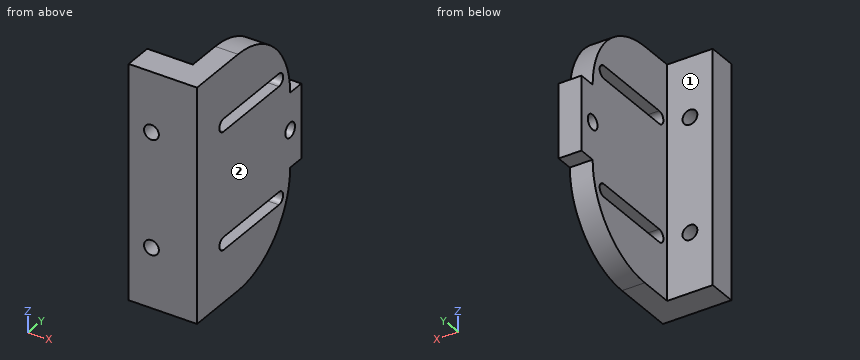
from build123d import *

# Parameters (mm, degrees)
SKETCH1_W           = 15.24
SKETCH1_H           = 52.07
BOSS_EXTRUDE1_DEPTH = 6.35
SKETCH2_W           = 5.08
SKETCH2_H           = 52.07
BOSS_EXTRUDE2_DEPTH = 25.4
CUT_EXTRUDE1_DEPTH  = 8.382
SKETCH4_R           = 1.651
CUT_EXTRUDE2_DEPTH  = 8.382
FILLET1_R           = 17.78
SKETCH6_W           = 5.08
SKETCH6_H           = 16.51
BOSS_EXTRUDE3_DEPTH = 3.81
SKETCH7_R           = 1.651
CUT_EXTRUDE3_DEPTH  = 14.478


with BuildPart() as part:
    # Sketch1 → Boss-Extrude1 (new body)
    with BuildSketch(Plane(origin=(0, 0, 0), x_dir=(1, 0, 0), z_dir=(0, 1, 0))):
        with Locations((7.62, 26.035)):
            Rectangle(SKETCH1_W, SKETCH1_H)
    extrude(amount=BOSS_EXTRUDE1_DEPTH)

    # Sketch2 → Boss-Extrude2 (add)
    with BuildSketch(Plane(origin=(0, 6.35, 0), x_dir=(1, 0, 0), z_dir=(0, 1, 0))):
        with Locations((12.7, 26.035)):
            Rectangle(SKETCH2_W, SKETCH2_H)
    extrude(amount=BOSS_EXTRUDE2_DEPTH)

    # Sketch3 → Cut-Extrude1 (cut)
    with BuildSketch(Plane(origin=(15.24, 0, 0), x_dir=(0, 0, -1), z_dir=(1, 0, 0))):
        with BuildLine():
            Line((14.4399, 27.94), (14.4399, 9.0424))
            ThreePointArc((14.4399, 9.0424), (13.0175, 7.62), (11.5951, 9.0424))
            Line((11.5951, 9.0424), (11.5951, 27.94))
            ThreePointArc((11.5951, 27.94), (13.0175, 29.3624), (14.4399, 27.94))
        make_face()
        with BuildLine():
            Line((40.50522627, 27.94), (40.50522627, 9.0424))
            ThreePointArc((40.50522627, 9.0424), (39.08282627, 7.62), (37.66042627, 9.0424))
            Line((37.66042627, 9.0424), (37.66042627, 27.94))
            ThreePointArc((37.66042627, 27.94), (39.08282627, 29.3624), (40.50522627, 27.94))
        make_face()
    extrude(amount=-CUT_EXTRUDE1_DEPTH, mode=Mode.SUBTRACT)

    # Sketch4 → Cut-Extrude2 (cut)
    with BuildSketch(Plane(origin=(0, 6.35, 0), x_dir=(1, 0, 0), z_dir=(0, 1, 0))):
        with Locations(Location((5.08, 38.735, 0), (0, 0, 270))):
            Circle(SKETCH4_R)
        with Locations(Location((5.08, 13.335, 0), (0, 0, 270))):
            Circle(SKETCH4_R)
    extrude(amount=-CUT_EXTRUDE2_DEPTH, mode=Mode.SUBTRACT)

    # Fillet1
    fillet1_edges = [part.edges().sort_by_distance(p)[0] for p in [
        (12.7, 31.75, -52.07),
        (12.7, 31.75, 0),
    ]]
    fillet(fillet1_edges, radius=FILLET1_R)

    # Sketch6 → Boss-Extrude3 (add)
    with BuildSketch(Plane(origin=(0, 31.75, 0), x_dir=(1, 0, 0), z_dir=(0, 1, 0))):
        with Locations((12.7, 26.035)):
            Rectangle(SKETCH6_W, SKETCH6_H)
    extrude(amount=BOSS_EXTRUDE3_DEPTH)

    # Sketch7 → Cut-Extrude3 (cut)
    with BuildSketch(Plane.ZY.offset(-10.16)):
        with Locations((-26.035, 31.75)):
            Circle(SKETCH7_R)
    extrude(amount=-CUT_EXTRUDE3_DEPTH, mode=Mode.SUBTRACT)


solid = part.part
Here's how the part is built. I have some questions about the finished solid (model axes, mm). Face numbers are marked on the shaded views. A direction names the side the tool comes from. Give positions to 0.01 mm unless a question says otherwise; leave off trailing zeros. Order: outer loops, then holes, each group sorted by start corner. A loop starts at its lowest first (then second) coordinate and runs counter-clockwise, first axis right, second up. Notation, with made-up numbers: (40.25, -1.75) -> (94.25, -1.75) arc R21 cw to (94.25, 32.25) -> close; hole circle Ø9 at (3, 57). An arc over 180 degrees is marked (long way). Use a Markdown table: item, result. Add a question column.
Item 1: Will these pins go through, and if not, where does the flat tip stop? pin 1 (5 mm diameter, centred on x = 2.5, z = -39.5, fed in from -Y); pin 2 (1.1 mm diameter, centred on x = 13.5, y = 33.5, fed in from +Z); pin 3 (1.1 mm diameter, centred on x = 13, y = 34, fed in from -Z); pin 4 (4 mm diameter, centred on x = 13, y = 21, fed in from +Z).
Item 2: Imagine slicing it at B-B on y = 20.5. Please give me the cut outline in (x, z).
Item 3: For the marked faces 1 and 2, which set-ups out of +Z, -Z, +X, -X, +Y, -Y let a thin tool reach every point of the face, with its end or its side?
Item 4: Imagine slicing it at D-D on x = 9. Please give me the cut outline in (y, z).
Item 5: Imagine slicing it at C-C on z = -28.5. Please give me the cut outline in (x, y).
Item 6: Imagine slicing it at A-A on x = 5.08. Please give me the cut outline in (y, z), plus the area to 3 significant figures.
Item 7: I need wall thicknesses on line 1 (Z direction, x = 10.25, y = 9); line 2 (Z direction, x = 13.25, y = 29); line 3 (X direction, y = 27, z = -27.5). Which ranges of each line are inside material? Lowest first, please.
Data:
| question | item | result |
|---|---|---|
| 1 | pin 1 | stops at y = 0 |
| 1 | pin 2 | stops at z = -17.78 |
| 1 | pin 3 | stops at z = -34.29 |
| 1 | pin 4 | stops at z = -0.73 |
| 2 | outline | (10.16, -50.83) -> (15.24, -50.83) -> (15.24, -40.51) -> (10.16, -40.51) -> close; (10.16, -37.66) -> (15.24, -37.66) -> (15.24, -14.44) -> (10.16, -14.44) -> close; (10.16, -11.6) -> (15.24, -11.6) -> (15.24, -1.24) -> (10.16, -1.24) -> close |
| 3 | face 1 | +Z, -Z, -X, +Y |
| 3 | face 2 | +Z, -Z, +X, +Y, -Y |
| 4 | outline | (0, -52.07) -> (6.35, -52.07) -> (6.35, 0) -> (0, 0) -> close |
| 5 | outline | (0, 0) -> (15.24, 0) -> (15.24, 35.56) -> (10.16, 35.56) -> (10.16, 6.35) -> (0, 6.35) -> close |
| 6 | outline | (0, -52.07) -> (6.35, -52.07) -> (6.35, -40.39) -> (0, -40.39) -> close; (0, -37.08) -> (6.35, -37.08) -> (6.35, -14.99) -> (0, -14.99) -> close; (0, -11.68) -> (6.35, -11.68) -> (6.35, 0) -> (0, 0) -> close |
| 6 | area | 289 mm² |
| 7 | line 1 | z = -52.07 to -40.5, -37.66 to -14.44, -11.6 to 0 |
| 7 | line 2 | z = -43.79 to -40.03, -38.13 to -13.97, -12.07 to -8.28 |
| 7 | line 3 | x = 10.16 to 15.24 |
